Check sheet for the drawn part. Datum: minimum x, y, z corner. Units: mm. Give positions to 0.01 mm unless a question says otherwise; leave off trailing zeros. Loops run counter-clockwise (first coordinate to the right, second up) from the corner with the lowest first, then second, coordinate; pieces in that order, holes last.
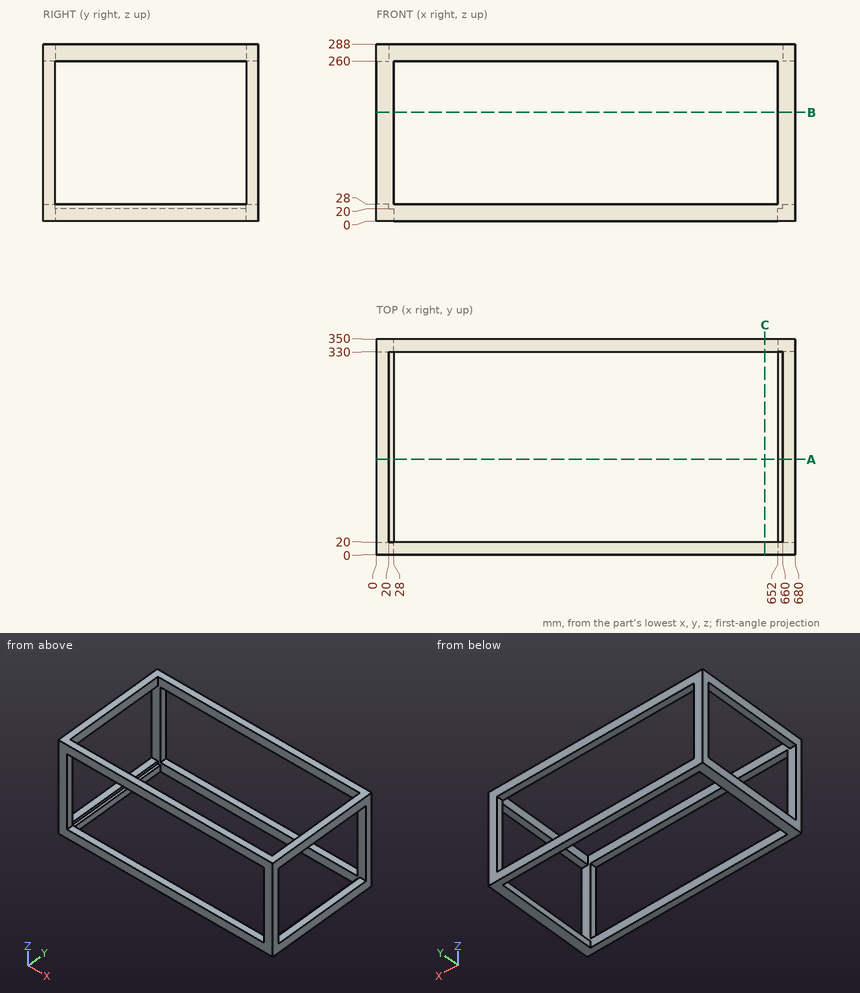
1) Sectioned sample at A-A on y = 155. Enter the section's corners in (x, z).
2) Sectioned sample at C-C on x = 631. Enter the section's corners in (y, z).
3) Sectioned sample at B-B on z = 177. Enter the section's corners in (x, y).
4) Scan lines: line 1 along Y through (x, z) = (467.5, 22.5); line 2 along X through (y, z) = (149, 264). Record each from-to range of solid material in increasing order.
Determined:
1. outline: (0, 0) - (28, 0) - (28, 20) - (20, 20) - (20, 28) - (0, 28) - close; (0, 260) - (20, 260) - (20, 288) - (0, 288) - close; (652, 0) - (680, 0) - (680, 28) - (660, 28) - (660, 20) - (652, 20) - close; (660, 260) - (680, 260) - (680, 288) - (660, 288) - close
2. outline: (0, 0) - (20, 0) - (20, 28) - (0, 28) - close; (0, 260) - (20, 260) - (20, 288) - (0, 288) - close; (330, 0) - (350, 0) - (350, 28) - (330, 28) - close; (330, 260) - (350, 260) - (350, 288) - (330, 288) - close
3. outline: (0, 0) - (28, 0) - (28, 20) - (0, 20) - close; (0, 330) - (28, 330) - (28, 350) - (0, 350) - close; (652, 0) - (680, 0) - (680, 20) - (652, 20) - close; (652, 330) - (680, 330) - (680, 350) - (652, 350) - close
4. line 1: y = 0 to 20, 330 to 350
4. line 2: x = 0 to 20, 660 to 680
